Could you check a few things on this model? Use its own coordinates, in mm. Give positions to 0.01 mm unless a question says otherwise; leave off trailing zeros. Order: outer loops, then holes, each group sorted by start corner. A loop starts at its lowest first (then second) coordinate and runs counter-clockwise, first axis right, second up. Notation, with made-up numbers: M 40.5,-39 L 60.5,-39 A19 ccw 60.5,-2 Z; hole C 75,27 d4. An arc over 180 degrees is marked long. Answer in a Markdown table with one row per item. Add a question column.
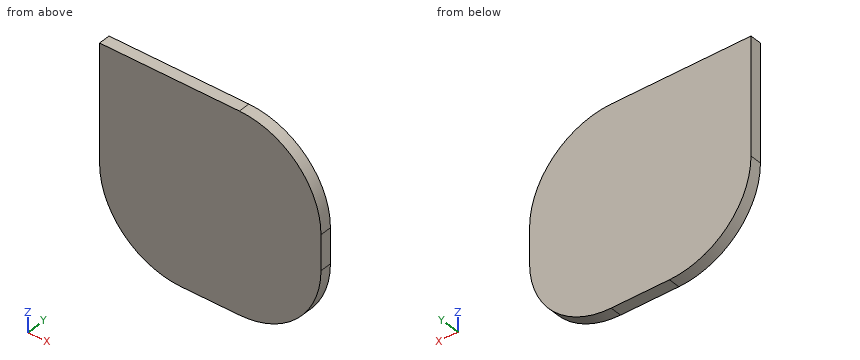
```python
from build123d import *

# Parameters (mm, degrees)
F0_W     = 48.26
F0_H     = 43.18
F1_DEPTH = 2.54
F2_R     = 17.78
F3_R     = 17.78


with BuildPart() as f1:
    # F0 (on Front) → F1 (new body)
    with BuildSketch(Plane.XZ):
        Rectangle(F0_W, F0_H)
    extrude(amount=F1_DEPTH)

    # F2
    f2_edges = [f1.edges().sort_by_distance(p)[0] for p in [
        (24.13, -1.27, -21.59),
        (-24.13, -1.27, -21.59),
    ]]
    fillet(f2_edges, radius=F2_R)

    # F3
    f3_edges = [f1.edges().sort_by_distance(p)[0] for p in [
        (24.13, -1.27, 21.59),
    ]]
    fillet(f3_edges, radius=F3_R)


solid = f1.part
```
1. Will this pin go through, and if not, where does the flat tip stop? P1, Ø3, axis at x = -15.5, z = 16.5, coming from the +Y side.
2. Suppose I cut it at A-A on y = -1.25. List the corners of the cut face in (x, z) for me.
3. Suppose I cut it at C-C on x = 12.5. List the corners of the cut face in (y, z) for me.
4. If I drill on line 1 along Z through (x, y) = (-6.5, -0.8); line 2 along Z through (x, y) = (21.5, -1.7); line 3 along X through (y, z) = (-1.3, 15.5), over which ranges is the centre line in solid material (lowest first)? Write a range as [from, to].
5. Suppose I cut it at B-B on z = 9. List the corners of the cut face in (x, y) for me, plus the area to 3 significant figures.
Findings below:
| question | item | result |
|---|---|---|
| 1 | P1 | y = 0 |
| 2 | outline | M -24.13,-3.81 A17.78 ccw -6.35,-21.59 L 6.35,-21.59 A17.78 ccw 24.13,-3.81 L 24.13,3.81 A17.78 ccw 6.35,21.59 L -24.13,21.59 Z |
| 3 | outline | M -2.54,-20.49 L 0,-20.49 L 0,20.49 L -2.54,20.49 Z |
| 4 | line 1 | [-21.59, 21.59] |
| 4 | line 2 | [-13.12, 13.12] |
| 4 | line 3 | [-24.13, 19.75] |
| 5 | outline | M -24.13,-2.54 L 23.36,-2.54 L 23.36,0 L -24.13,0 Z |
| 5 | area | 121 mm2 |
